Verification items for the finished model (mm, model axes). Round coordinates to 2 decimals unless told otherwise and drop trailing zeros. Write each loop counter-clockwise with the first axis right and the second up, starting at its lowest first coordinate (ties: lowest second). Pieces come first, ordered by that corner, then holes. Notation, with made-up numbers: (12.5, 50.25) - (57.5, 50.25) arc R18 cw to (57.5, 76.25) - close; hole circle Ø7 at (65, -4.75). An arc over 180 degrees is marked (long way). Answer as a JSON object with one key per item and string values. Group by question number.
1) Mould release check, pull along Z, two halves, no side actions. Record for faces 1 (the flat face through (51, 2, -173)), 2 (the flat face through (65, 1, -88)), 3 (the conical face through (34.807, 1.681, -29.314)): +Z half, -Z half, draft (parallel to the pull), parting line (faces both ways), or undercut.
2) Section check A-A (y = 0.35). State how many separate pieces and enclosed holes the cut face has, then the cut area to 3 significant figures.
3) Section check C-C (x = 53). Enter the section's corners in (y, z), then the cut area to 3 significant figures.
4) Section check B-B (x = 76). Enter the section's corners in (y, z).
5) Go/stop test with flat-tipped pins: pin 1 Ø4 at (x, z) = (-16.09, -160.04) entering from -Y; pin 2 Ø2.5 at (x, z) = (30.95, -159.3) entering from -Y; pin 3 Ø0.6 at (y, z) = (0.5, -308) entering from +X; pin 4 Ø3.5 at (x, z) = (18.97, -256.93) entering from -Y. Record where each tip stops, or that it passes through.
6) Thickness scan on line 1 (Z direction, x = 9, y = 0.7); line 2 (Z direction, x = 23.5, y = 1); line 3 (X direction, y = 0.15, z = -182.5). Record the ranges inside material, lowest first.
```python
from build123d import *

# Parameters (mm, degrees)
BOSS_EXTRUDE2_DEPTH = 2
SKETCH5_W           = 23
SKETCH5_H           = 26
CUT_EXTRUDE1_DEPTH  = 2
SKETCH6_W           = 23
SKETCH6_H           = 26
CUT_EXTRUDE2_DEPTH  = 2
SKETCH7_W           = 12
SKETCH7_H           = 20
CUT_EXTRUDE3_DEPTH  = 2
SKETCH8_W           = 12
SKETCH8_H           = 20
CUT_EXTRUDE4_DEPTH  = 2
SKETCH9_R           = 1.5
CUT_EXTRUDE5_DEPTH  = 4
SKETCH10_R          = 1.5
CUT_EXTRUDE6_DEPTH  = 4
SKETCH11_R          = 1.5
SKETCH11_R_2        = 1.556495296
CUT_EXTRUDE7_DEPTH  = 4
CHAMFER1_SIZE       = 2
SKETCH12_W          = 41.427208619
SKETCH12_H          = 13.04809718
CUT_EXTRUDE8_DEPTH  = 4
SKETCH13_R          = 1.5
CUT_EXTRUDE9_DEPTH  = 10
CHAMFER2_SIZE       = 2
SKETCH14_W          = 23
SKETCH14_H          = 3.896287967
BOSS_EXTRUDE3_DEPTH = 2
SKETCH15_W          = 23
SKETCH15_H          = 6.016100964
CUT_EXTRUDE10_DEPTH = 2
SKETCH16_W          = 23
SKETCH16_H          = 4.189884345
CUT_EXTRUDE11_DEPTH = 2
SKETCH17_R          = 1.5
CUT_EXTRUDE12_DEPTH = 2
CHAMFER4_SIZE       = 2
SKETCH19_W          = 23
SKETCH19_H          = 7.922215634
CUT_EXTRUDE13_DEPTH = 2
SKETCH20_W          = 23
SKETCH20_H          = 2.611384529
CUT_EXTRUDE14_DEPTH = 2
SKETCH22_W          = 23
SKETCH22_H          = 5.13756828
BOSS_EXTRUDE5_DEPTH = 2
SKETCH23_R          = 1.5
CUT_EXTRUDE16_DEPTH = 2
CHAMFER6_SIZE       = 2
SKETCH24_R          = 1.5
CUT_EXTRUDE17_DEPTH = 10
CHAMFER7_SIZE       = 1
CUT_EXTRUDE18_REACH = 352.962
SKETCH25_R          = 1.5
CHAMFER8_SIZE       = 1


# Some blends are built 0.0001 mm under size
with BuildPart() as part:
    # Sketch4 → Boss-Extrude2 (new body)
    with BuildSketch(Plane(origin=(0, 0, 0), x_dir=(1, 0, 0), z_dir=(0, 1, 0))):
        Polygon((0, 341), (0, 276), (-36, 276), (-36, 110), (0, 66), (0, 0), (47, 0), (47, 66), (83, 110), (83, 276), (47, 276), (47, 341), align=None)
    extrude(amount=BOSS_EXTRUDE2_DEPTH)

    # Sketch5 → Cut-Extrude1 (cut)
    with BuildSketch(Plane(origin=(0, 2, 0), x_dir=(1, 0, 0), z_dir=(0, 1, 0))):
        with Locations((23.5, 42)):
            Rectangle(SKETCH5_W, SKETCH5_H)
    extrude(amount=-CUT_EXTRUDE1_DEPTH, mode=Mode.SUBTRACT)

    # Sketch6 → Cut-Extrude2 (cut)
    with BuildSketch(Plane(origin=(0, 2, 0), x_dir=(1, 0, 0), z_dir=(0, 1, 0))):
        with Locations((23.5, 299)):
            Rectangle(SKETCH6_W, SKETCH6_H)
    extrude(amount=-CUT_EXTRUDE2_DEPTH, mode=Mode.SUBTRACT)

    # Sketch7 → Cut-Extrude3 (cut)
    with BuildSketch(Plane(origin=(0, 2, 0), x_dir=(1, 0, 0), z_dir=(0, 1, 0))):
        with Locations((-21, 242)):
            Rectangle(SKETCH7_W, SKETCH7_H)
    extrude(amount=-CUT_EXTRUDE3_DEPTH, mode=Mode.SUBTRACT)

    # Sketch8 → Cut-Extrude4 (cut)
    with BuildSketch(Plane(origin=(0, 2, 0), x_dir=(1, 0, 0), z_dir=(0, 1, 0))):
        with Locations((10, 242)):
            Rectangle(SKETCH8_W, SKETCH8_H)
    extrude(amount=-CUT_EXTRUDE4_DEPTH, mode=Mode.SUBTRACT)

    # Sketch9 → Cut-Extrude5 (cut)
    with BuildSketch(Plane(origin=(0, 2, 0), x_dir=(1, 0, 0), z_dir=(0, 1, 0))):
        with Locations(Location((-9.668146344, 96.299430829, 0), (0, 0, 270))):
            Circle(SKETCH9_R)
        with Locations(Location((60.331853656, 96.299430845, 0), (0, 0, 270))):
            Circle(SKETCH9_R)
    extrude(amount=-CUT_EXTRUDE5_DEPTH, mode=Mode.SUBTRACT)

    # Sketch10 → Cut-Extrude6 (cut)
    with BuildSketch(Plane(origin=(0, 2, 0), x_dir=(1, 0, 0), z_dir=(0, 1, 0))):
        with Locations(Location((45.515605611, 272, 0), (0, 0, 270))):
            Circle(SKETCH10_R)
        with Locations(Location((45.515605611, 203, 0), (0, 0, 270))):
            Circle(SKETCH10_R)
    extrude(amount=-CUT_EXTRUDE6_DEPTH, mode=Mode.SUBTRACT)

    # Sketch11 → Cut-Extrude7 (cut)
    with BuildSketch(Plane(origin=(0, 2, 0), x_dir=(1, 0, 0), z_dir=(0, 1, 0))):
        with Locations(Location((27.453567096, 192.29943079, 0), (0, 0, 270))):
            Circle(SKETCH11_R)
        with Locations(Location((16.999402189, 192.117575161, 0), (0, 0, 270))):
            Circle(SKETCH11_R_2)
        with Locations(Location((12.953567087, 159.299430834, 0), (0, 0, 270))):
            Circle(SKETCH11_R)
        with Locations(Location((30.953567087, 159.299430838, 0), (0, 0, 270))):
            Circle(SKETCH11_R)
    extrude(amount=-CUT_EXTRUDE7_DEPTH, mode=Mode.SUBTRACT)

    # Chamfer1
    chamfer1_edges = [part.edges().sort_by_distance(p)[0] for p in [
        (-9.668146344, 0, -97.799430829),
        (60.331853656, 0, -97.799430845),
        (45.515605611, 0, -273.5),
        (45.515605611, 0, -204.5),
        (30.953567087, 0, -160.799430838),
        (12.953567087, 0, -160.799430834),
        (16.999402189, 0, -193.674070457),
        (27.453567096, 0, -193.79943079),
    ]]
    chamfer(chamfer1_edges, length=CHAMFER1_SIZE - 0.0001)  # a hair under: the kernel refuses the full size

    # Sketch12 → Cut-Extrude8 (cut)
    with BuildSketch(Plane(origin=(0, 2, 0), x_dir=(1, 0, 0), z_dir=(0, 1, 0))):
        with Locations((21.45416489, 176.373831134)):
            Rectangle(SKETCH12_W, SKETCH12_H)
    extrude(amount=-CUT_EXTRUDE8_DEPTH, mode=Mode.SUBTRACT)

    # Sketch13 → Cut-Extrude9 (cut)
    with BuildSketch(Plane(origin=(0, 2, 0), x_dir=(1, 0, 0), z_dir=(0, 1, 0))):
        with Locations(Location((-16.085510492, 160.04183924, 0), (0, 0, 270))):
            Circle(SKETCH13_R)
        with Locations(Location((-10.282531236, 121.164739857, 0), (0, 0, 270))):
            Circle(SKETCH13_R)
    extrude(amount=-CUT_EXTRUDE9_DEPTH, mode=Mode.SUBTRACT)

    # Chamfer2
    chamfer2_edges = [part.edges().sort_by_distance(p)[0] for p in [
        (-16.085510492, 0, -161.54183924),
        (-10.282531236, 0, -122.664739857),
    ]]
    chamfer(chamfer2_edges, length=CHAMFER2_SIZE - 0.0001)  # a hair under: the kernel refuses the full size

    # Sketch14 → Boss-Extrude3 (add)
    with BuildSketch(Plane(origin=(0, 0, 0), x_dir=(-1, 0, 0), z_dir=(0, -1, 0))):
        with Locations((-23.5, 30.948143984)):
            Rectangle(SKETCH14_W, SKETCH14_H)
    extrude(amount=-BOSS_EXTRUDE3_DEPTH)

    # Sketch15 → Cut-Extrude10 (cut)
    with BuildSketch(Plane.XZ):
        with Locations((23.5, -58.008050482)):
            Rectangle(SKETCH15_W, SKETCH15_H)
    extrude(amount=-CUT_EXTRUDE10_DEPTH, mode=Mode.SUBTRACT)

    # Sketch16 → Cut-Extrude11 (cut)
    with BuildSketch(Plane.XZ):
        with Locations((23.5, -63.111043137)):
            Rectangle(SKETCH16_W, SKETCH16_H)
    extrude(amount=-CUT_EXTRUDE11_DEPTH, mode=Mode.SUBTRACT)

    # Sketch17 → Cut-Extrude12 (cut)
    with BuildSketch(Plane(origin=(0, 2, 0), x_dir=(1, 0, 0), z_dir=(0, 1, 0))):
        with Locations(Location((34.01068775, 76.54942652, 0), (0, 0, 270))):
            Circle(SKETCH17_R)
        with Locations(Location((12.76068775, 76.549426515, 0), (0, 0, 270))):
            Circle(SKETCH17_R)
        with Locations(Location((12.760687761, 31.049426515, 0), (0, 0, 270))):
            Circle(SKETCH17_R)
        with Locations(Location((34.260687761, 31.04942652, 0), (0, 0, 270))):
            Circle(SKETCH17_R)
    extrude(amount=-CUT_EXTRUDE12_DEPTH, mode=Mode.SUBTRACT)

    # Chamfer4
    # the kernel refuses this chamfer: 2 mm, written as the material it takes off along each edge
    with BuildSketch(Plane(origin=(34.260687761, 0, -31.04942652), x_dir=(0, 0, 1), z_dir=(-1, 0, 0))) as chamfer4_piece_1:
        Polygon((1.5 + CHAMFER4_SIZE, 0), (1.5, CHAMFER4_SIZE), (1.5, 0), align=None)
    revolve(axis=Axis((34.260687761, 0, -31.04942652), (0, 1, 0)), mode=Mode.SUBTRACT)
    with BuildSketch(Plane(origin=(12.760687761, 0, -31.049426515), x_dir=(0, 0, 1), z_dir=(-1, 0, 0))) as chamfer4_piece_2:
        Polygon((1.5 + CHAMFER4_SIZE, 0), (1.5, CHAMFER4_SIZE), (1.5, 0), align=None)
    revolve(axis=Axis((12.760687761, 0, -31.049426515), (0, 1, 0)), mode=Mode.SUBTRACT)
    with BuildSketch(Plane(origin=(12.76068775, 0, -76.549426515), x_dir=(0, 0, 1), z_dir=(-1, 0, 0))) as chamfer4_piece_3:
        Polygon((1.5 + CHAMFER4_SIZE, 0), (1.5, CHAMFER4_SIZE), (1.5, 0), align=None)
    revolve(axis=Axis((12.76068775, 0, -76.549426515), (0, 1, 0)), mode=Mode.SUBTRACT)
    with BuildSketch(Plane(origin=(34.01068775, 0, -76.54942652), x_dir=(0, 0, 1), z_dir=(-1, 0, 0))) as chamfer4_piece_4:
        Polygon((1.5 + CHAMFER4_SIZE, 0), (1.5, CHAMFER4_SIZE), (1.5, 0), align=None)
    revolve(axis=Axis((34.01068775, 0, -76.54942652), (0, 1, 0)), mode=Mode.SUBTRACT)

    # Sketch19 → Cut-Extrude13 (cut)
    with BuildSketch(Plane.XZ):
        with Locations((23.5, -315.961107817)):
            Rectangle(SKETCH19_W, SKETCH19_H)
    extrude(amount=-CUT_EXTRUDE13_DEPTH, mode=Mode.SUBTRACT)

    # Sketch20 → Cut-Extrude14 (cut)
    with BuildSketch(Plane.XZ):
        with Locations((23.5, -321.227907899)):
            Rectangle(SKETCH20_W, SKETCH20_H)
    extrude(amount=-CUT_EXTRUDE14_DEPTH, mode=Mode.SUBTRACT)

    # Sketch22 → Boss-Extrude5 (add)
    with BuildSketch(Plane(origin=(0, 0, 0), x_dir=(-1, 0, 0), z_dir=(0, -1, 0))):
        with Locations((-23.5, 288.56878414)):
            Rectangle(SKETCH22_W, SKETCH22_H)
    extrude(amount=-BOSS_EXTRUDE5_DEPTH)

    # Sketch23 → Cut-Extrude16 (cut)
    with BuildSketch(Plane(origin=(0, 2, 0), x_dir=(1, 0, 0), z_dir=(0, 1, 0))):
        with Locations(Location((12.74123696, 334.049079093, 0), (0, 0, 270))):
            Circle(SKETCH23_R)
        with Locations(Location((34.24123696, 334.049079093, 0), (0, 0, 270))):
            Circle(SKETCH23_R)
        with Locations(Location((34.24123696, 288.549079093, 0), (0, 0, 270))):
            Circle(SKETCH23_R)
        with Locations(Location((12.74123696, 288.549079093, 0), (0, 0, 270))):
            Circle(SKETCH23_R)
    extrude(amount=-CUT_EXTRUDE16_DEPTH, mode=Mode.SUBTRACT)

    # Chamfer6
    # the kernel refuses this chamfer: 2 mm, written as the material it takes off along each edge
    with BuildSketch(Plane(origin=(12.74123696, 0, -288.549079093), x_dir=(0, 0, 1), z_dir=(-1, 0, 0))) as chamfer6_piece_1:
        Polygon((1.5 + CHAMFER6_SIZE, 0), (1.5, CHAMFER6_SIZE), (1.5, 0), align=None)
    revolve(axis=Axis((12.74123696, 0, -288.549079093), (0, 1, 0)), mode=Mode.SUBTRACT)
    with BuildSketch(Plane(origin=(34.24123696, 0, -288.549079093), x_dir=(0, 0, 1), z_dir=(-1, 0, 0))) as chamfer6_piece_2:
        Polygon((1.5 + CHAMFER6_SIZE, 0), (1.5, CHAMFER6_SIZE), (1.5, 0), align=None)
    revolve(axis=Axis((34.24123696, 0, -288.549079093), (0, 1, 0)), mode=Mode.SUBTRACT)
    with BuildSketch(Plane(origin=(34.24123696, 0, -334.049079093), x_dir=(0, 0, 1), z_dir=(-1, 0, 0))) as chamfer6_piece_3:
        Polygon((1.5 + CHAMFER6_SIZE, 0), (1.5, CHAMFER6_SIZE), (1.5, 0), align=None)
    revolve(axis=Axis((34.24123696, 0, -334.049079093), (0, 1, 0)), mode=Mode.SUBTRACT)
    with BuildSketch(Plane(origin=(12.74123696, 0, -334.049079093), x_dir=(0, 0, 1), z_dir=(-1, 0, 0))) as chamfer6_piece_4:
        Polygon((1.5 + CHAMFER6_SIZE, 0), (1.5, CHAMFER6_SIZE), (1.5, 0), align=None)
    revolve(axis=Axis((12.74123696, 0, -334.049079093), (0, 1, 0)), mode=Mode.SUBTRACT)

    # Sketch24 → Cut-Extrude17 (cut)
    with BuildSketch(Plane(origin=(0, 2, 0), x_dir=(1, 0, 0), z_dir=(0, 1, 0))):
        with Locations(Location((-31.031546179, 256.928363681, 0), (0, 0, 270))):
            Circle(SKETCH24_R)
        with Locations(Location((-31.031546172, 224.928363681, 0), (0, 0, 270))):
            Circle(SKETCH24_R)
        with Locations(Location((18.968453821, 256.928363693, 0), (0, 0, 270))):
            Circle(SKETCH24_R)
        with Locations(Location((18.968453828, 224.928363693, 0), (0, 0, 270))):
            Circle(SKETCH24_R)
    extrude(amount=-CUT_EXTRUDE17_DEPTH, mode=Mode.SUBTRACT)

    # Chamfer7
    chamfer7_edges = [part.edges().sort_by_distance(p)[0] for p in [
        (-31.031546172, 0, -226.428363681),
        (18.968453821, 0, -258.428363693),
        (18.968453828, 0, -226.428363693),
        (-31.031546179, 0, -258.428363681),
    ]]
    chamfer(chamfer7_edges, length=CHAMFER7_SIZE)

    # Sketch25 → Cut-Extrude18 (cut, up to next)
    with BuildSketch(Plane.XZ, mode=Mode.PRIVATE) as cut_extrude18_sk1:
        with Locations(Location((14.087342161, -7.092513938, 0), (0, 0, 270))):
            Circle(SKETCH25_R)
    cut_extrude18_tool1 = extrude(cut_extrude18_sk1.sketch, amount=-CUT_EXTRUDE18_REACH, mode=Mode.PRIVATE) & part.part
    # Sketch25 → Cut-Extrude18 (cut, up to next)
    with BuildSketch(Plane.XZ, mode=Mode.PRIVATE) as cut_extrude18_sk2:
        with Locations(Location((34.087342161, -7.092513938, 0), (0, 0, 270))):
            Circle(SKETCH25_R)
    cut_extrude18_tool2 = extrude(cut_extrude18_sk2.sketch, amount=-CUT_EXTRUDE18_REACH, mode=Mode.PRIVATE) & part.part
    add(cut_extrude18_tool1.solids().sort_by_distance((14.087342, 0, -7.092514))[0], mode=Mode.SUBTRACT)
    add(cut_extrude18_tool2.solids().sort_by_distance((34.087342, 0, -7.092514))[0], mode=Mode.SUBTRACT)

    # Chamfer8
    chamfer8_edges = [part.edges().sort_by_distance(p)[0] for p in [
        (14.087342161, 2, -5.592513938),
        (34.087342161, 2, -5.592513938),
    ]]
    chamfer(chamfer8_edges, length=CHAMFER8_SIZE)


solid = part.part
```
Returned:
{
 "1": {"face 1": "draft", "face 2": "+Z half", "face 3": "undercut"},
 "2": {"separate pieces": "1", "enclosed holes": "25", "area": "26,500 mm2"},
 "3": {"outline": "(0, -276) - (2, -276) - (2, -73.33) - (0, -73.33) - close", "area": "405 mm2"},
 "4": {"outline": "(0, -276) - (2, -276) - (2, -101.44) - (0, -101.44) - close"},
 "5": {"pin 1": "y = 1.5", "pin 2": "through", "pin 3": "x = 47", "pin 4": "y = 0.75"},
 "6": {"line 1": "-341 to -252, -232 to -182.9, -169.85 to 0", "line 2": "-341 to -322.53, -291.14 to -182.9, -169.85 to -65.21, -32.9 to 0", "line 3": "-36 to 0.74, 42.17 to 83"}
}
